Design review of the part built by this model. Coordinates are the model's own, in mm. A direction names the side the tool comes from. Coordinates: 2 decimals unless noted, no trailing zeros. Loops run counter-clockwise (first coordinate to the right, second up) from the corner with the lowest first, then second, coordinate; pieces in that order, holes last. Notation, with made-up numbers: (-5, 20) -> (50, 20) arc R21 cw to (50, 38) -> close; hole circle Ø1 at (75, -13.75). An arc over 180 degrees is marked (long way). Answer in a Markdown table with one row per item.
```python
from build123d import *

# Parameters (mm, degrees)
SKETCH1_W           = 57.15
SKETCH1_H           = 25.4
BOSS_EXTRUDE1_DEPTH = 6.35
SKETCH2_W           = 19.05
SKETCH2_H           = 12.7
BOSS_EXTRUDE2_DEPTH = 6.35
FILLET1_R           = 0.508


with BuildPart() as part:
    # Sketch1 → Boss-Extrude1 (new, symmetric)
    with BuildSketch(Plane(origin=(0, 0, 0), x_dir=(1, 0, 0), z_dir=(0, 1, 0))):
        Rectangle(SKETCH1_W, SKETCH1_H)
    extrude(amount=BOSS_EXTRUDE1_DEPTH, both=True)

    # Sketch2 → Boss-Extrude2 (add)
    with BuildSketch(Plane.XY.offset(12.7)):
        with Locations((19.05, 0)):
            Rectangle(SKETCH2_W, SKETCH2_H)
    extrude(amount=BOSS_EXTRUDE2_DEPTH)

    # Fillet1
    fillet1_edges = [part.edges().sort_by_distance(p)[0] for p in [
        (-9.525, 6.35, 12.7),
        (-9.525, -6.35, 12.7),
    ]]
    fillet(fillet1_edges, radius=FILLET1_R)


solid = part.part
```
(1) Take a section at C-C on z = 14.5. Give the boundary of the cut face in (x, y) (3 decimals), and give its area (3 significant figures).
Evaluation:
| item | result |
|---|---|
| outline | (9.525, -6.35) -> (28.575, -6.35) -> (28.575, 6.35) -> (9.525, 6.35) -> close |
| area | 242 mm² |
(2) To check wall thickness, follow probe 1 along X at (y, z) = (-1.25, 13) (3 decimals); probe 2 along Z at (x, y) = (-8, 2.5); probe 3 along Z at (x, y) = (-5, 6.25). State the ranges of each line that lie inside material, in increasing order.
Evaluation:
| item | result |
|---|---|
| probe 1 | x = 9.525 to 28.575 |
| probe 2 | z = -12.7 to 12.7 |
| probe 3 | z = -12.7 to 12.49 |
(3) Tool access review of faces 1 (the flat face through (-10, 0, 12.7)), 2 (the flat face through (19, 0, 19.05)): name each direction out of +Z, -Z, +X, -X, +Y, -Y from which nothing blocks a thin tool from reaching the whole face with its end or side.
Evaluation:
| item | result |
|---|---|
| face 1 | +Z, -X, +Y, -Y |
| face 2 | +Z, +X, -X, +Y, -Y |
(4) Take a section at B-B on x = -21.5. Give the boundary of the cut face in (y, z), and give its area (3 significant figures).
Evaluation:
| item | result |
|---|---|
| outline | (-6.35, -12.7) -> (6.35, -12.7) -> (6.35, 12.19) arc R0.51 ccw to (5.84, 12.7) -> (-5.84, 12.7) arc R0.51 ccw to (-6.35, 12.19) -> close |
| area | 322 mm² |
(5) Take a section at A-A on y = 4. Give the boundary of the cut face in (x, z) (3 decimals).
Evaluation:
| item | result |
|---|---|
| outline | (-28.575, -12.7) -> (28.575, -12.7) -> (28.575, 19.05) -> (9.525, 19.05) -> (9.525, 12.7) -> (-28.575, 12.7) -> close |
(6) For pin 1 (1.5 mm diameter, centred on x = 2, y = -1.5, fed in from +Z), flat-tipped, find the tip position at first contact; note if it passes through.
Evaluation:
| item | result |
|---|---|
| pin 1 | stops at z = 12.7 |
